Can you work these out from the model? Positions are in its coordinate system, mm. A direction names the side the tool comes from. Coordinates: 2 decimals unless noted, no trailing zeros. Loops run counter-clockwise (first coordinate to the right, second up) from the corner with the lowest first, then second, coordinate; pieces in that order, holes last. Notation, with made-up numbers: (11.5, 24.5) -> (15.5, 24.5) arc R11 ccw to (15.5, 38.5) -> close; hole circle Ø6 at (-26, 55). An arc over 180 degrees is marked (long way). Use one line per item in the form item = value. Start each with the question number.
(1) Imagine slicing it at A-A (x = 16). List the corners of the cut face in (y, z) for me, plus the area to 3 significant figures.
(2) Imagine slicing it at D-D (y = 7.75). List the corners of the cut face in (x, z) for me, plus the area to 3 significant figures.
(3) I need wall thicknesses on line 1 (Z direction, x = -12.5, y = -1.5); line 2 (Y direction, x = -18.5, z = -2.5); line 3 (Y direction, x = -19, z = 21.5). Which ranges of each line are inside material? Lowest first, please. Write a range as [from, to].
(4) Thinking about a two-plate mould opening in Z: for faces 4 (the flat face through (-25, 0, 5)), 5 (the flat face through (-8, 2, 23.438)), 6 (the flat face through (-11.22, 7.479, 3.604)), which applies, released by +Z, released by -Z, zero draft, split by the parting line, or undercut?
(5) Imagine slicing it at C-C (z = 14). List the corners of the cut face in (x, y) for me.
(6) Imagine slicing it at B-B (y = 2.5). List the corners of the cut face in (x, z) for me, plus the area to 3 significant figures.
(7) On a 3-axis mill with a long thin cutter (end or side, diameter ignored), from which of +Z, -Z, +X, -X, +Y, -Y can I reach the whole of each face in a straight line? I mean faces 1 (the flat face through (-3.098, 7, 6)), 2 (the cylindrical face through (21.7, -1.5, 0)), 3 (the flat face through (-6, 0, -4.562)). Say none if no direction works.
(8) I'm going to push flat-ended pins straight in: pin 1 (2 mm diameter, centred on x = -13, z = 3.5, fed in from -Y); pin 2 (2.5 mm diameter, centred on x = -25.85, z = 0.44, fed in from -Y); pin 3 (15 mm diameter, centred on x = 17.5, z = 1, fed in from +Y); pin 4 (12 mm diameter, centred on y = 11, z = 0.5, fed in from -X). Where does each tip first touch, or does it pass through?
```python
from build123d import *

# Parameters (mm, degrees)
SKETCH1_W           = 8
SKETCH1_H           = 20
SKETCH1_W_2         = 56
SKETCH1_H_2         = 8
BOSS_EXTRUDE1_DEPTH = 3
SKETCH2_W           = 18
SKETCH2_H           = 8
BOSS_EXTRUDE2_DEPTH = 6
SKETCH3_W           = 18
SKETCH3_H           = 36
BOSS_EXTRUDE3_DEPTH = 5.3
SKETCH5_R           = 1.9
CUT_EXTRUDE1_DEPTH  = 5.3
SKETCH6_R           = 3
SKETCH6_R_2         = 1.9
BOSS_EXTRUDE5_DEPTH = 9
CUT_EXTRUDE2_DEPTH  = 3
SKETCH8_R           = 2
CUT_EXTRUDE3_DEPTH  = 3


with BuildPart() as part:
    # Sketch1 → Boss-Extrude1 (new body)
    with BuildSketch(Plane(origin=(0, 0, 0), x_dir=(1, 0, 0), z_dir=(0, 1, 0))):
        Polygon((-29.097818748, 12.561692374), (-29.097818748, 4.561692374), (-21.097818748, 4.561692374), (18.902181252, 4.561692374), (26.902181252, 4.561692374), (26.902181252, 12.561692374), align=None)
        with Locations((-25.097818748, -5.438307626)):
            Rectangle(SKETCH1_W, SKETCH1_H)
        with Locations((22.902181252, -5.438307626)):
            Rectangle(SKETCH1_W, SKETCH1_H)
        with Locations((-1.097818748, -19.438307626)):
            Rectangle(SKETCH1_W_2, SKETCH1_H_2)
    extrude(amount=-BOSS_EXTRUDE1_DEPTH)

    # Sketch2 → Boss-Extrude2 (add)
    with BuildSketch(Plane(origin=(0, 0, 0), x_dir=(1, 0, 0), z_dir=(0, 1, 0))):
        with Locations((-12.097818748, 8.561692374)):
            Rectangle(SKETCH2_W, SKETCH2_H)
        with Locations((-12.097818748, -19.438307626)):
            Rectangle(SKETCH2_W, SKETCH2_H)
    extrude(amount=BOSS_EXTRUDE2_DEPTH)

    # Sketch3 → Boss-Extrude3 (add)
    with BuildSketch(Plane(origin=(0, 6, 0), x_dir=(1, 0, 0), z_dir=(0, 1, 0))):
        with Locations((-12.097818748, -5.438307626)):
            Rectangle(SKETCH3_W, SKETCH3_H)
    extrude(amount=BOSS_EXTRUDE3_DEPTH)

    # Sketch5 → Cut-Extrude1 (cut)
    with BuildSketch(Plane(origin=(0, 6, 0), x_dir=(1, 0, 0), z_dir=(0, 1, 0))):
        with Locations(Location((-14.097818748, -5.438307626, 0), (0, 0, 270))):
            Circle(SKETCH5_R)
    extrude(amount=CUT_EXTRUDE1_DEPTH, mode=Mode.SUBTRACT)

    # Sketch6 → Boss-Extrude5 (add)
    with BuildSketch(Plane(origin=(0, 11.3, 0), x_dir=(1, 0, 0), z_dir=(0, 1, 0))):
        with Locations(Location((-14.097818748, -5.438307626, 0), (0, 0, 90))):
            Circle(SKETCH6_R)
        with Locations(Location((-14.097818748, -5.438307626, 0), (0, 0, 270))):
            Circle(SKETCH6_R_2, mode=Mode.SUBTRACT)
    extrude(amount=BOSS_EXTRUDE5_DEPTH)

    # Sketch7 → Cut-Extrude2 (cut)
    with BuildSketch(Plane.XZ.offset(-6)):
        Polygon((-12.250616402, 1.957625885), (-10.159858765, 5.297690913), (-12.00706111, 8.778372654), (-15.945021093, 8.918989367), (-18.03577873, 5.578924339), (-16.188576385, 2.098242598), align=None)
    extrude(amount=-CUT_EXTRUDE2_DEPTH, mode=Mode.SUBTRACT)

    # Sketch8 → Cut-Extrude3 (cut)
    with BuildSketch(Plane(origin=(0, 0, 0), x_dir=(1, 0, 0), z_dir=(0, 1, 0))):
        with Locations(Location((23.652181252, -0.438307626, 0), (0, 0, 270))):
            Circle(SKETCH8_R)
        with Locations(Location((23.652181252, -10.438307626, 0), (0, 0, 270))):
            Circle(SKETCH8_R)
        with Locations(Location((-25.847818748, -0.438307626, 0), (0, 0, 270))):
            Circle(SKETCH8_R)
        with Locations(Location((-25.847818748, -10.438307626, 0), (0, 0, 270))):
            Circle(SKETCH8_R)
    extrude(amount=-CUT_EXTRUDE3_DEPTH, mode=Mode.SUBTRACT)


solid = part.part
```
Worked out:
q1.outline = (-3, -12.56) -> (0, -12.56) -> (0, -4.56) -> (-3, -4.56) -> close; (-3, 15.44) -> (0, 15.44) -> (0, 23.44) -> (-3, 23.44) -> close
q1.area = 48.0 mm2
q2.outline = (-21.1, -12.56) -> (-3.1, -12.56) -> (-3.1, 23.44) -> (-21.1, 23.44) -> close; hole (-18.04, 5.58) -> (-16.19, 2.1) -> (-12.25, 1.96) -> (-10.16, 5.3) -> (-12.01, 8.78) -> (-15.95, 8.92) -> close
q2.area = 608 mm2
q3.line_1 = [-12.56, -4.56], [15.44, 23.44]
q3.line_2 = [6, 11.3]
q3.line_3 = [-3, 11.3]
q4.face_4 = zero draft
q4.face_5 = released by +Z
q4.face_6 = undercut
q5.outline = (-29.1, -3) -> (-21.1, -3) -> (-21.1, 0) -> (-29.1, 0) -> close; (-21.1, 6) -> (-3.1, 6) -> (-3.1, 11.3) -> (-21.1, 11.3) -> close; (18.9, -3) -> (26.9, -3) -> (26.9, 0) -> (18.9, 0) -> close
q6.outline = (-21.1, -12.56) -> (-3.1, -12.56) -> (-3.1, -4.56) -> (-21.1, -4.56) -> close; (-21.1, 15.44) -> (-3.1, 15.44) -> (-3.1, 23.44) -> (-21.1, 23.44) -> close
q6.area = 288 mm2
q7.face_1 = +Z, -Z, +X, +Y
q7.face_2 = +Y, -Y
q7.face_3 = -Y
q8.pin_1 = 9
q8.pin_2 = through
q8.pin_3 = 0
q8.pin_4 = -21.1
